Build history of the part. All positions in model axes, mm. Face numbers are marked on the shaded views. A direction names the side the tool comes from. Round coordinates to 2 decimals unless told otherwise and drop trailing zeros. Order: outer loops, then holes, each group sorted by start corner. A loop starts at its lowest first (then second) coordinate and runs counter-clockwise, first axis right, second up. Notation, with made-up numbers: (-10.5, 67.5) -> (35.5, 67.5) arc R20 ccw to (35.5, 80.5) -> close; hole circle Ø1 at (6, -31.75). An arc over 180 degrees is marked (long way). Use a Markdown table: item, result. Add a question column.
Item 1: 3-axis set-ups, long thin cutter, end or side, ignore diameter. For the marked faces 1 and 2: which of +Z, -Z, +X, -X, +Y, -Y reach the whole face in a straight line?
Item 2: Slice it at A-A, the plane y = -2. Give the cut face in (x, z) (3 decimals), plus the area to 3 significant figures.
Item 3: Pin check, flat tips, straight feed: pin 1 (1 mm diameter, centred on y = -4, z = -1.5, fed in from -X); pin 2 (1.4 mm diameter, centred on x = 0, z = 0, fed in from -Y); pin 3 (4 mm diameter, centred on x = 34, y = 1.5, fed in from +Z); pin 4 (1.5 mm diameter, centred on x = 18, z = -0.5, fed in from -Y). Stop position of each tip, or through.
Item 4: Probe L1, parallel to X at y = -3.5, z = 0 (3 decimals); L2, parallel to Y at x = 40, z = 0.25; L3, parallel to Z at x = -1.5, y = -1.5 (3 decimals). List the from-to ranges inside material, lowest first.
from build123d import *

# Parameters (mm, degrees)
BOSS_EXTRUDE1_DEPTH = 3
FILLET1_SIZE        = 2
FILLET1_SIZE_2      = 5
SKETCH2_R           = 1.875
SKETCH2_R_2         = 0.875
BOSS_EXTRUDE3_DEPTH = 9
CUT_EXTRUDE2_START  = -0.5
SKETCH4_R           = 0.875
CUT_EXTRUDE2_DEPTH  = 43.942490853


with BuildPart() as part:
    # Sketch1 → Boss-Extrude1 (new body)
    with BuildSketch(Plane(origin=(0, 0, 0), x_dir=(1, 0, 0), z_dir=(0, 1, 0))):
        with BuildLine():
            Line((0, 6.5), (42, 6.5))
            Line((42, 6.5), (42, -6.5))
            Line((42, -6.5), (0, -6.5))
            ThreePointArc((0, -6.5), (-6.5, 0), (0, 6.5))
        make_face()
    extrude(amount=BOSS_EXTRUDE1_DEPTH)

    # Fillet1
    # an asymmetric fillet: 5, 2 mm, written as the material it takes off along each edge
    with BuildSketch(Plane(origin=(0, 0, -6.5), x_dir=(0, 1, 0), z_dir=(1, 0, 0)), Plane(origin=(54.5, 0, 6.5), x_dir=(0, 1, 0), z_dir=(-1, 0, 0))) as fillet1_piece_1:
        with BuildLine():
            Bezier((FILLET1_SIZE, 0), (0, 0), (0, FILLET1_SIZE_2), weights=[1, 0.707106781, 1])
            Line((0, FILLET1_SIZE_2), (0, 0))
            Line((0, 0), (FILLET1_SIZE, 0))
        make_face()
    extrude(amount=54.5, mode=Mode.SUBTRACT)
    with BuildSketch(Plane(origin=(0, 0, 0), x_dir=(0, 0, 1), z_dir=(1, 0, 0))) as fillet1_piece_2:
        with BuildLine():
            Bezier((6.5, -FILLET1_SIZE), (6.5, 0), (6.5 - FILLET1_SIZE_2, 0), weights=[1, 0.707106781, 1])
            Line((6.5 - FILLET1_SIZE_2, 0), (6.5, 0))
            Line((6.5, 0), (6.5, -FILLET1_SIZE))
        make_face()
    revolve(axis=Axis((0, 0, 0), (0, -1, 0)), revolution_arc=180, mode=Mode.SUBTRACT)

    # Sketch2 → Boss-Extrude3 (add)
    with BuildSketch(Plane(origin=(0, 3, 0), x_dir=(1, 0, 0), z_dir=(0, 1, 0))):
        with Locations(Location((0, 0, 0), (0, 0, 270))):
            Circle(SKETCH2_R)
        with Locations(Location((0, 0, 0), (0, 0, 270))):
            Circle(SKETCH2_R_2, mode=Mode.SUBTRACT)
    extrude(amount=-BOSS_EXTRUDE3_DEPTH)

    # Sketch4 → Cut-Extrude2 (cut, through all)
    with BuildSketch(Plane(origin=(0, 3, 0), x_dir=(1, 0, 0), z_dir=(0, 1, 0)).offset(CUT_EXTRUDE2_START)):
        with Locations(Location((0, 0, 0), (0, 0, 270))):
            Circle(SKETCH4_R)
    extrude(amount=-CUT_EXTRUDE2_DEPTH, mode=Mode.SUBTRACT)


solid = part.part
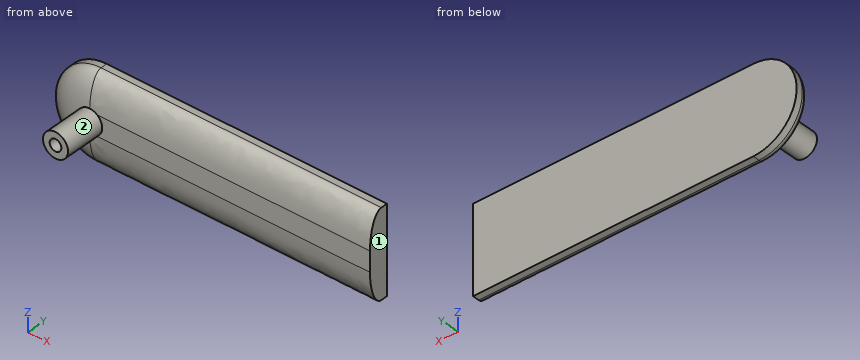
Check sheet entries:
| question | item | result |
|---|---|---|
| 1 | face 1 | +Z, -Z, +X, +Y, -Y |
| 1 | face 2 | -Y |
| 2 | outline | circle Ø3.75 at (0, 0); hole circle Ø1.75 at (0, 0) |
| 2 | area | 8.64 mm2 |
| 3 | pin 1 | x = -1.59 |
| 3 | pin 2 | y = 2.5 |
| 3 | pin 3 | z = 6.5 |
| 3 | pin 4 | y = 0 |
| 4 | L1 | -1.875 to -0.875, 0.875 to 1.875 |
| 4 | L2 | 0 to 3 |
| 4 | L3 | -1.125 to 1.125 |
